The model under review builds one solid part; all positions refer to its coordinate system, in mm. A direction names the side the tool comes from. Round coordinates to 2 decimals unless told otherwise and drop trailing zeros. Write each loop counter-clockwise with the first axis right and the second up, starting at its lowest first coordinate (ties: lowest second). Pieces come first, ordered by that corner, then holes.
Item 1: Add section D-D (x = 7.25). Give the boundary of the cut face in (y, z).
Item 2: Add section C-C (y = 29.5). Give the boundary of the cut face in (x, z).
Item 3: Clearance check with flat-ended pins moving along their axes: pin 1 Ø1.5 at (y, z) = (17.5, 0) entering from -X; pin 2 Ø6 at (y, z) = (25.5, 1.5) entering from +X; pin 3 Ø1.5 at (x, y) = (3, 22.5) entering from +Z. State where each tip first meets the part, or that it passes through.
Item 4: Add section B-B (y = 24). Give the boundary of the cut face in (x, z).
Item 5: Add section A-A (z = 0). Give the boundary of the cut face in (x, y), plus the area to 4 significant figures.
Item 6: Machinability: for faces 4 (the face through (1.46, 9.42, 6.59)), 5 (the face through (2, 21, -6)), 6 (the face through (5, 20, 0)), 7 (the face through (2, 21, 6)), which of the approach directions +Z, -Z, +X, -X, +Y, -Y give a long, thin tool a straight path to every point of the face, cutting with its end or side? Answer none if there is none.
Item 7: Draft analysis for pull direction Z (two halves, no side actions). For faces 1 (the face through (2.5, 22.8, 2.4)), 2 (the face through (-2, 16, 0)), 3 (the face through (-6.1, 1.1, 1.9)), state which applies: +Z half, -Z half, draft (parallel to the pull), parting line (faces both ways), or undercut.
Item 8: To check wall thickness, follow L1, parallel to Z at x = 3.5, y = 26; L2, parallel to Z at x = -0.25, y = 6; L3, parallel to Y at x = 2.5, z = -1.75. State the ranges of each line that lie inside material, in increasing order.
Autodesk Inventor part; units mm, degrees
ref_plane "YZ Plane" through (0, 0, 0) normal (1, 0, 0) x (0, 1, 0)
ref_plane "XZ Plane" through (0, 0, 0) normal (0, 1, 0) x (-1, 0, 0)
ref_plane "XY Plane" through (0, 0, 0) normal (0, 0, 1) x (1, 0, 0)
sketch "Sketch1" plane through (0, 0, 0) normal (0, 1, 0) x (-1, 0, 0)
  circle A0 centre (0, 0) radius 6.75
  dimension "d0" = 13.5
extrude "Extrusion1" add sketch "Sketch1" along normal blind 15
chamfer "Chamfer1" distance 4 distance2 0.5 1 edges at (6.75, 0, 0) measured on face at (-6.7281, 10, -0.5431)
sketch "Sketch2" plane through (0, 15, 0) normal (0, 1, 0) x (1, 0, 0)
  circle A0 centre (0, 0) radius 8
  dimension "d6" = 16
extrude "Extrusion2" add sketch "Sketch2" along normal blind 1
sketch "Sketch3" plane through (0, 0, 0) normal (1, 0, 0) x (0, 1, 0)
  circle A0 centre (26, 0) radius 4
  arc A1 (26, -6) -> (26, 6) centre (26, 0) ccw
  line L0 (16, -8) -> (16, 8)
  line L1 (26, 6) -> (16, 6)
  line L2 (16, 6) -> (16, -6)
  line L3 (16, -6) -> (26, -6)
  point P0 (0, 0)
  dimension "d9" = 8
  dimension "d10" = 2
  dimension "d11" = 10
extrude "Extrusion3" add sketch "Sketch3" along normal blind 5
properties part number "center_holder_top"
Numbers:
1. outline: (15, -3.38) - (16, -3.38) - (16, 3.38) - (15, 3.38) - close
2. outline: (0, -4.87) - (5, -4.87) - (5, -1.94) - (0, -1.94) - close; (0, 1.94) - (5, 1.94) - (5, 4.87) - (0, 4.87) - close
3. pin 1: stops at x = 0
3. pin 2: stops at x = 5
3. pin 3: stops at z = 6
4. outline: (0, -6) - (5, -6) - (5, -3.46) - (0, -3.46) - close; (0, 3.46) - (5, 3.46) - (5, 6) - (0, 6) - close
5. outline: (-8, 15) - (-6.75, 15) - (-6.75, 4) - (-6.25, 0) - (6.25, 0) - (6.75, 4) - (6.75, 15) - (8, 15) - (8, 16) - (5, 16) - (5, 22) - (0, 22) - (0, 16) - (-8, 16) - close; (0, 30) - (5, 30) - (5, 32) - (0, 32) - close
5. area: 256.5 mm2
6. face 4: -Y
6. face 5: -Z, +X, -X, +Y
6. face 6: +Z, -Z, +X, +Y
6. face 7: +Z, +X, -X, +Y
7. face 1: undercut
7. face 2: draft
7. face 3: parting line
8. L1: z = -6 to -4, 4 to 6
8. L2: z = -6.75 to 6.75
8. L3: y = 0 to 22.4, 29.6 to 31.74
